```python
from build123d import *

# Parameters (mm, degrees)
SKETCH2_R                                     = 47.5
BOSS_EXTRUDE2_DEPTH                           = 100
SKETCH3_R                                     = 44.5
CUT_EXTRUDE1_DEPTH                            = 97
SKETCH4_W                                     = 145.572703988
SKETCH4_H                                     = 25
SKETCH4_W_2                                   = 159.095851353
CUT_EXTRUDE3_DEPTH                            = 95
BOSS_EXTRUDE3_DEPTH                           = 5
FILLET1_R                                     = 5
CBORE_FOR_3_SOCKET_HEAD_CAP_SCREW1_AT_2_COUNT = 2
CBORE_FOR_3_SOCKET_HEAD_CAP_SCREW1_AT_2_PITCH = 116.131492307
BOSS_EXTRUDE4_DEPTH                           = 45
SKETCH10_W                                    = 9
SKETCH10_H                                    = 14
CUT_EXTRUDE4_DEPTH                            = 43
SKETCH11_W                                    = 15
SKETCH11_H                                    = 8
CUT_EXTRUDE5_DEPTH                            = 4
SKETCH12_W                                    = 15
SKETCH12_H                                    = 8
CUT_EXTRUDE6_DEPTH                            = 4
CUT_EXTRUDE7_REACH                            = 169.726
CUT_EXTRUDE7_END_RADIUS                       = 44.5
SKETCH13_R                                    = 3.15
CUT_EXTRUDE8_REACH                            = 161.839
CUT_EXTRUDE8_END_RADIUS                       = 44.5
SKETCH14_R                                    = 2.65


with BuildPart() as part:
    # Sketch2 → Boss-Extrude2 (new body)
    with BuildSketch(Plane(origin=(0, 0, 0), x_dir=(1, 0, 0), z_dir=(0, 1, 0))):
        with Locations(Location((0, 0, 0), (0, 0, 270))):
            Circle(SKETCH2_R)
    extrude(amount=BOSS_EXTRUDE2_DEPTH)

    # Sketch3 → Cut-Extrude1 (cut)
    with BuildSketch(Plane(origin=(0, 100, 0), x_dir=(1, 0, 0), z_dir=(0, 1, 0))):
        with Locations(Location((0, 0, 0), (0, 0, 270))):
            Circle(SKETCH3_R)
    extrude(amount=-CUT_EXTRUDE1_DEPTH, mode=Mode.SUBTRACT)

    # Sketch4 → Cut-Extrude3 (cut)
    with BuildSketch(Plane(origin=(0, 100, 0), x_dir=(1, 0, 0), z_dir=(0, 1, 0))):
        with Locations((2.391411924, -22.5)):
            Rectangle(SKETCH4_W, SKETCH4_H)
        with Locations((9.152985607, 22.5)):
            Rectangle(SKETCH4_W_2, SKETCH4_H)
    extrude(amount=-CUT_EXTRUDE3_DEPTH, mode=Mode.SUBTRACT)

    # Sketch5 → Boss-Extrude3 (add)
    with BuildSketch(Plane.XZ):
        with BuildLine():
            Line((-9.162255845, 46.607972149), (-9.162255845, 55.903490308))
            ThreePointArc((-9.162255845, 55.903490308), (0, 65.065746153), (9.162255845, 55.903490308))
            Line((9.162255845, 55.903490308), (9.162255845, 46.607972149))
            ThreePointArc((9.162255845, 46.607972149), (0, 47.5), (-9.162255845, 46.607972149))
        make_face()
        with BuildLine():
            Line((9.162255845, -46.607972149), (9.162255845, -55.903490308))
            ThreePointArc((9.162255845, -55.903490308), (0, -65.065746153), (-9.162255845, -55.903490308))
            Line((-9.162255845, -55.903490308), (-9.162255845, -46.607972149))
            ThreePointArc((-9.162255845, -46.607972149), (0, -47.5), (9.162255845, -46.607972149))
        make_face()
    extrude(amount=-BOSS_EXTRUDE3_DEPTH)

    # Fillet1
    fillet1_edges = [part.edges().sort_by_distance(p)[0] for p in [
        (0, 5, -47.5),
        (4.602788445, 5, 47.276467069),
    ]]
    fillet(fillet1_edges, radius=FILLET1_R)

    # Sketch8 → CBORE for #3 Socket Head Cap Screw1 (revolve, cut)
    with BuildSketch(Plane(origin=(0, 5, 58.065746153), x_dir=(0, 0, 1), z_dir=(1, 0, 0))):
        Polygon((0, 0), (0, 5), (1.397, 5), (1.397, 2.5146), (2.57937, 2.5146), (2.57937, 0.635), (3.21437, 0), align=None)
    cbore_for_3_socket_head_cap_screw1 = revolve(axis=Axis((0, 11.35, 58.065746153), (0, -1, 0)), mode=Mode.SUBTRACT)

    # CBORE for #3 Socket Head Cap Screw1 at 2: CBORE for #3 Socket Head Cap Screw1 ×2
    with Locations(*[(0, 0, -i * CBORE_FOR_3_SOCKET_HEAD_CAP_SCREW1_AT_2_PITCH) for i in range(1, CBORE_FOR_3_SOCKET_HEAD_CAP_SCREW1_AT_2_COUNT)]):
        add(cbore_for_3_socket_head_cap_screw1, mode=Mode.SUBTRACT)

    # Sketch9 → Boss-Extrude4 (add)
    with BuildSketch(Plane.XZ):
        with BuildLine():
            Line((-58.325612467, 10), (-46.435439053, 10))
            ThreePointArc((-46.435439053, 10), (-47.5, 0), (-46.435439053, -10))
            Line((-46.435439053, -10), (-58.325612467, -10))
            Line((-58.325612467, -10), (-58.325612467, 10))
        make_face()
        with BuildLine():
            Line((46.435439053, 10), (59.566582945, 10))
            Line((59.566582945, 10), (59.566582945, -10))
            Line((59.566582945, -10), (46.435439053, -10))
            ThreePointArc((46.435439053, -10), (47.5, 0), (46.435439053, 10))
        make_face()
    extrude(amount=-BOSS_EXTRUDE4_DEPTH)

    # Sketch10 → Cut-Extrude4 (cut)
    with BuildSketch(Plane.XZ):
        with Locations((-51.602219379, 0.189273316)):
            Rectangle(SKETCH10_W, SKETCH10_H)
        with Locations((52.545961871, 0.189273316)):
            Rectangle(SKETCH10_W, SKETCH10_H)
    extrude(amount=-CUT_EXTRUDE4_DEPTH, mode=Mode.SUBTRACT)

    # Sketch11 → Cut-Extrude5 (cut)
    with BuildSketch(Plane(origin=(59.566582945, 0, 0), x_dir=(0, 0, -1), z_dir=(1, 0, 0))):
        with Locations((-0.034463617, 37)):
            Rectangle(SKETCH11_W, SKETCH11_H)
    extrude(amount=-CUT_EXTRUDE5_DEPTH, mode=Mode.SUBTRACT)

    # Sketch12 → Cut-Extrude6 (cut)
    with BuildSketch(Plane.ZY.offset(58.325612467)):
        with Locations((0.376507126, 37)):
            Rectangle(SKETCH12_W, SKETCH12_H)
    extrude(amount=-CUT_EXTRUDE6_DEPTH, mode=Mode.SUBTRACT)

    # Cut-Extrude7: up to this cylinder (the profile starts outside it)
    cut_extrude7_end = Plane(origin=(0, 36.5, 0), z_dir=(0, 1, 0)) * Cylinder(CUT_EXTRUDE7_END_RADIUS, 429.452, mode=Mode.PRIVATE)
    # Sketch13 → Cut-Extrude7 (cut, up to the surface)
    with BuildSketch(Plane.ZY.offset(58.325612467), mode=Mode.PRIVATE) as cut_extrude7_sk1:
        with Locations((0, 36.5)):
            Circle(SKETCH13_R)
    cut_extrude7_tool1 = extrude(cut_extrude7_sk1.sketch, amount=-CUT_EXTRUDE7_REACH, mode=Mode.PRIVATE) - cut_extrude7_end
    add(cut_extrude7_tool1.solids().sort_by_distance((-58.325612, 36.5, 0))[0], mode=Mode.SUBTRACT)

    # Cut-Extrude8: up to this cylinder (the profile starts outside it)
    cut_extrude8_end = Plane(origin=(0, 36.5, 0), z_dir=(0, 1, 0)) * Cylinder(CUT_EXTRUDE8_END_RADIUS, 413.678, mode=Mode.PRIVATE)
    # Sketch14 → Cut-Extrude8 (cut, up to the surface)
    with BuildSketch(Plane(origin=(48.045961871, 0, 0), x_dir=(0, 0, -1), z_dir=(1, 0, 0)), mode=Mode.PRIVATE) as cut_extrude8_sk1:
        with Locations((0, 36.5)):
            Circle(SKETCH14_R)
    cut_extrude8_tool1 = extrude(cut_extrude8_sk1.sketch, amount=-CUT_EXTRUDE8_REACH, mode=Mode.PRIVATE) - cut_extrude8_end
    add(cut_extrude8_tool1.solids().sort_by_distance((48.045962, 36.5, 0))[0], mode=Mode.SUBTRACT)


solid = part.part
```
Source: CAD feature listing. Evaluate the final solid. Frame: model axes, mm. A direction names the side the tool comes from. Round coordinates to 2 decimals unless told otherwise and drop trailing zeros. Loops run counter-clockwise (first coordinate to the right, second up) from the corner with the lowest first, then second, coordinate; pieces in that order, holes last. Notation, with made-up numbers: M 5.5,33 L 18.5,33 A24 ccw 18.5,58 Z; hole C -9.5,-13 d7. An arc over 180 degrees is marked long. Use a Markdown table: item, result. Add a question column.
1. Cut plane A-A, the plane y = 13. Output: boundary loops of the cut face in (x, z), and give its area (3 significant figures).
2. Cut plane D-D, the plane x = -39.5. Output: boundary loops of the cut face in (y, z), and give its area (3 significant figures).
3. Cut plane C-C, the plane z = 0. State how many separate pieces and enclosed holes the cut face has, and give its area (3 significant figures).
4. Pull-direction query (Z, two-part tool) for faces 1 (the cylindrical face through (-47.5, 72.1, -0.1)), 2 (the cylindrical face through (0.201, 2.465, -65.064)), 3 (the flat face through (58, 41, 0)), 4 (the flat face through (58, 37, 7.534)); classes: +Z half, -Z half, draft (parallel to the pull), parting line (faces both ways), or undercut.
5. Cut plane B-B, the plane y = 62.5. Output: boundary loops of the cut face in (x, z), and give its area (3 significant figures).
6. Contact query for flat-ended pins moving along their axis: pin 1 (1.5 mm diameter, centred on x = 0.5, z = 59, fed in from +Y); pin 2 (1.5 mm diameter, centred on x = 8, y = 70.5, fed in from -Z); pin 3 (5 mm diameter, centred on x = 54, y = 27, fed in from +Z); pin 4 (10 mm diameter, centred on x = 30.5, z = 46.5, fed in from +Y). Output: stop coordinate, or through.
7. Set-up query: faces 5 (the flat face through (38.3, 5, -23.5)), 6 (the flat face through (-52, 21, -6.811)). Return all of +Z, -Z, +X, -X, +Y, -Y with unobstructed straight access to the full face (end or side cutting, diameter ignored); none if empty.
8. Ray query, line 1 along Y through (x, z) = (-45.7, 0); line 2 along Y through (x, z) = (45.55, 0); line 3 along Z through (x, y) = (0, 92). Return the intervals inside material, ascending. Write a range as [from, to].
Solution:
| question | item | result |
|---|---|---|
| 1 | outline | M -58.33,-10 L -43.36,-10 A44.5 cw -43.36,10 L -58.33,10 Z; M -32.11,-35 A47.5 ccw 32.11,-35 L 27.48,-35 A44.5 cw -27.48,-35 Z; M -32.11,35 L -27.48,35 A44.5 cw 27.48,35 L 32.11,35 A47.5 ccw Z; M 43.36,-10 L 59.57,-10 L 59.57,10 L 43.36,10 A44.5 cw Z; hole M -56.1,-6.81 L -47.1,-6.81 L -47.1,7.19 L -56.1,7.19 Z; hole M 48.05,-6.81 L 57.05,-6.81 L 57.05,7.19 L 48.05,7.19 Z |
| 1 | area | 731 mm2 |
| 2 | outline | M 0,-26.38 L 5,-26.38 L 5,-20.49 L 3,-20.49 L 3,20.49 L 5,20.49 L 5,26.38 L 0,26.38 Z |
| 2 | area | 182 mm2 |
| 3 | separate pieces | 5 |
| 3 | enclosed holes | 0 |
| 3 | area | 1,050 mm2 |
| 4 | face 1 | parting line |
| 4 | face 2 | -Z half |
| 4 | face 3 | undercut |
| 4 | face 4 | undercut |
| 5 | outline | M -46.44,-10 L -43.36,-10 A44.5 cw -43.36,10 L -46.44,10 A47.5 ccw Z; M -32.11,-35 A47.5 ccw 32.11,-35 L 27.48,-35 A44.5 cw -27.48,-35 Z; M -32.11,35 L -27.48,35 A44.5 cw 27.48,35 L 32.11,35 A47.5 ccw Z; M 43.36,-10 L 46.44,-10 A47.5 ccw 46.44,10 L 43.36,10 A44.5 cw Z |
| 5 | area | 511 mm2 |
| 6 | pin 1 | stops at y = 2.49 |
| 6 | pin 2 | stops at z = -46.94 |
| 6 | pin 3 | stops at z = 10 |
| 6 | pin 4 | passes through |
| 7 | face 5 | +X, -X, +Y |
| 7 | face 6 | -Y |
| 8 | line 1 | y = [0, 33.35], [39.65, 100] |
| 8 | line 2 | y = [0, 33.85], [39.15, 100] |
| 8 | line 3 | z = [-47.5, -44.5], [44.5, 47.5] |
